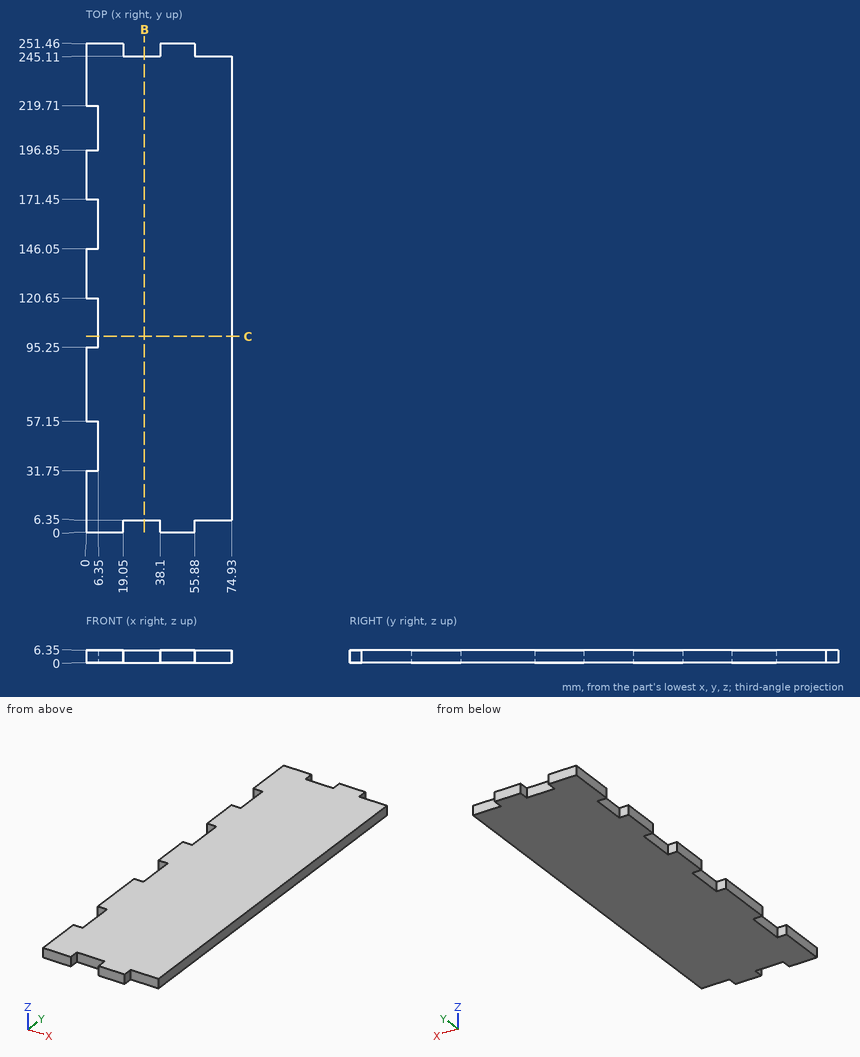
Input: dimensioned drawing with shaded views. Units: mm. Origin: part minimum x, y, z. Coordinates: 2 decimals unless noted, no trailing zeros. Order: outer loops, then holes, each group sorted by start corner. A loop starts at its lowest first (then second) coordinate and runs counter-clockwise, first axis right, second up. Notation, with made-up numbers: (84.5, 87) - (98.5, 87) arc R8 ccw to (98.5, 94) - close; hole circle Ø1 at (55, -28). An arc over 180 degrees is marked (long way). Put each result on its own line as item: value.
1. Cut plane B-B on x = 30. Return the cut outline in (y, z).
Report:
outline: (6.35, 0) - (245.11, 0) - (245.11, 6.35) - (6.35, 6.35) - close
2. Contact query for flat-ended pins moving along their axis: pin 1 Ø3 at (x, z) = (33, 2.5) entering from +Y; pin 2 Ø3 at (y, z) = (160, 2) entering from -X; pin 3 Ø3 at (y, z) = (2.5, 1.5) entering from +X. Output: stop coordinate, or through.
Report:
pin 1: stops at y = 245.11
pin 2: stops at x = 6.35
pin 3: stops at x = 55.88
3. Line query: line 1 along Y through (x, z) = (31, 6); line 2 along X through (y, z) = (204, 5.75). Output: solid intervals per line, ascending.
Report:
line 1: y = 6.35 to 245.11
line 2: x = 6.35 to 74.93
4. Cut plane C-C on y = 101. Return the cut outline in (x, z), then the cut area to 3 significant figures.
Report:
outline: (6.35, 0) - (74.93, 0) - (74.93, 6.35) - (6.35, 6.35) - close
area: 435 mm2
